Part model, mm, in its own coordinate system. Coordinates: 2 decimals unless noted, no trailing zeros. Write each loop counter-clockwise with the first axis right and the second up, starting at its lowest first coordinate (ties: lowest second). Pieces come first, ordered by that corner, then holes. Notation, with made-up numbers: (74.5, 10) -> (116.5, 10) arc R27 ccw to (116.5, 26) -> close; hole circle Ø5 at (-37, 82). An arc over 180 degrees is marked (long way). One line per question, with ' | ' between items. Start each with the question number.
Item 1: Two-plate mould, pull along X, no slides. Class faces 1 (the cylindrical face through (12.122, -374.384, 2.504)), 2 (the cylindrical face through (-19.57, -376.4, 2.5)), 3 (the cylindrical face through (0.97, -439, 2.5)): pulls with the +X half, pulls with the -X half, needs draft (parallel to the pull), parting line crosses it, or undercut.
Item 2: Pin check, flat tips, straight feed: pin 1 (1 mm diameter, centred on y = -423, z = 0.5, fed in from +X); pin 2 (1 mm diameter, centred on x = 17, z = 4.5, fed in from -Y). Stop position of each tip, or through.
Item 3: Saw through at B-B (x = 12). List the corners of the cut face in (y, z).
Item 4: Saw through at C-C (y = -391). List the corners of the cut face in (x, z), and give its area (3 significant figures).
Item 5: Saw through at D-D (x = 27). List the corners of the cut face in (y, z).
Item 6: Saw through at A-A (z = 1.9). List the corners of the cut face in (x, y), and give its area (3 significant figures).
Item 7: Probe probe 1 along X at (y, z) = (-374.5, 4.1); probe 2 along Y at (x, z) = (-9, 2.15); probe 3 along Y at (x, z) = (12, 0.55). List the from-to ranges inside material, lowest first. Write a range as [from, to].
from build123d import *

# Parameters (mm, degrees)
SKETCH1_R           = 2.54
BOSS_EXTRUDE1_DEPTH = 5.08


with BuildPart() as part:
    # Sketch1 → Boss-Extrude1 (new body)
    with BuildSketch(Plane.XY):
        with BuildLine():
            Line((-16.923532905, -361.932719801), (16.923532905, -361.932719801))
            ThreePointArc((16.923532905, -361.932719801), (19.506243092, -376.204363349), (26.016534546, -389.164544931))
            ThreePointArc((26.016534546, -389.164544931), (0, -439.01304823), (-26.016534546, -389.164544931))
            ThreePointArc((-26.016534546, -389.164544931), (-19.506243092, -376.204363349), (-16.923532905, -361.932719801))
        make_face()
        with Locations((-10.756405179, -376.525575709)):
            Circle(SKETCH1_R, mode=Mode.SUBTRACT)
        with Locations((10.756405179, -376.525575709)):
            Circle(SKETCH1_R, mode=Mode.SUBTRACT)
    extrude(amount=BOSS_EXTRUDE1_DEPTH)


solid = part.part
From the geometry:
1) face 1: undercut | face 2: pulls with the -X half | face 3: parting line crosses it
2) pin 1: x = 27.83 | pin 2: y = -434.38
3) outline: (-436.66, 0) -> (-378.74, 0) -> (-378.74, 5.08) -> (-436.66, 5.08) -> close; (-374.31, 0) -> (-361.93, 0) -> (-361.93, 5.08) -> (-374.31, 5.08) -> close
4) outline: (-27.2, 0) -> (27.2, 0) -> (27.2, 5.08) -> (-27.2, 5.08) -> close | area: 276 mm2
5) outline: (-423.94, 0) -> (-390.66, 0) -> (-390.66, 5.08) -> (-423.94, 5.08) -> close
6) outline: (-26.02, -389.16) arc R31.71 ccw (long way) to (26.02, -389.16) arc R50.8 cw to (16.92, -361.93) -> (-16.92, -361.93) arc R50.8 cw to start; hole circle Ø5.08 at (-10.76, -376.53); hole circle Ø5.08 at (10.76, -376.53) | area: 3,710 mm2
7) probe 1: [-18.97, -12.29], [-9.22, 9.22], [12.29, 18.97] | probe 2: [-437.71, -378.36], [-374.69, -361.93] | probe 3: [-436.66, -378.74], [-374.31, -361.93]
